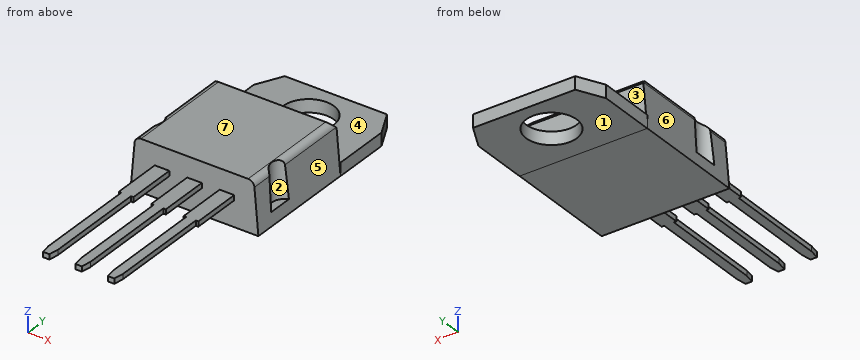
```python
from build123d import *

# Parameters (mm, degrees)
SKETCH2_W                = 10
SKETCH2_H                = 9
BOSS_EXTRUDE1_DEPTH      = 4
CHAMFER1_SIZE            = 0.5
CUT_EXTRUDE1_DEPTH       = 3
BOSS_EXTRUDE2_DEPTH      = 0.4
LPATTERN1_COUNT          = 2
LPATTERN1_PITCH          = 2.54
LPATTERN2_COUNT          = 2
LPATTERN2_PITCH          = 2.54
DRAFT2_ANGLE             = -5
BOSS_EXTRUDE3_DEPTH      = 0.01
BOSS_EXTRUDE3_DEPTH_BACK = 1
SKETCH8_R                = 1.98
FILLET1_R                = 0.5
SCALE1_SCALE             = 0.6


with BuildPart() as part:
    # Sketch2 → Boss-Extrude1 (new body)
    with BuildSketch(Plane.XY):
        Rectangle(SKETCH2_W, SKETCH2_H)
    extrude(amount=BOSS_EXTRUDE1_DEPTH)

    # Chamfer1
    chamfer1_edges = [part.edges().sort_by_distance(p)[0] for p in [
        (0, 4.5, 4),
    ]]
    chamfer(chamfer1_edges, length=CHAMFER1_SIZE)

    # Sketch6 → Cut-Extrude1 (cut)
    with BuildSketch(Plane.XY.offset(4)):
        with BuildLine():
            Line((5, -1), (5, -3))
            ThreePointArc((5, -3), (4.25, -2), (5, -1))
        make_face()
    cut_extrude1 = extrude(amount=-CUT_EXTRUDE1_DEPTH, mode=Mode.SUBTRACT)

    # Mirror1: Cut-Extrude1 across plane
    add(cut_extrude1.mirror(Plane(origin=(0, 0, 0), x_dir=(0, 0, 1), z_dir=(1, 0, 0))), mode=Mode.SUBTRACT)

    # Sketch7 → Boss-Extrude2 (add)
    with BuildSketch(Plane.XY.offset(2)):
        Polygon((-0.57, -4.5), (-0.57, -8.44), (-0.375, -8.44), (-0.375, -16.44), (-0.25, -17.2), (0.25, -17.2), (0.375, -16.44), (0.375, -8.44), (0.57, -8.44), (0.57, -4.5), align=None)
    boss_extrude2 = extrude(amount=BOSS_EXTRUDE2_DEPTH)

    # LPattern1: Boss-Extrude2 ×2
    with Locations(*[(-i * LPATTERN1_PITCH, 0, 0) for i in range(1, LPATTERN1_COUNT)]):
        add(boss_extrude2)

    # LPattern2: Boss-Extrude2 ×2
    with Locations(*[(i * LPATTERN2_PITCH, 0, 0) for i in range(1, LPATTERN2_COUNT)]):
        add(boss_extrude2)

    # Draft2
    draft2_faces = [part.faces().sort_by_distance(p)[0] for p in [
        (5, 0.383542538, 1.891910739),
        (-5, 0.383542538, 1.891910739),
    ]]
    draft(draft2_faces, Plane(origin=(0, 0, 0), x_dir=(-1, 0, 0), z_dir=(0, 0, -1)), DRAFT2_ANGLE)

    # Sketch8 → Boss-Extrude3 (add, two sides: drawn at the far end of the back side and taken through both)
    with BuildSketch(Plane(origin=(0, 0, 0), x_dir=(-1, 0, 0), z_dir=(0, 0, -1)).offset(-BOSS_EXTRUDE3_DEPTH_BACK)):
        Polygon((-5, 9), (-4, 11), (4, 11), (5, 9), (5, 4.5), (-5, 4.5), align=None)
        with Locations(Location((0, 8, 0), (0, 0, 180))):
            Circle(SKETCH8_R, mode=Mode.SUBTRACT)
    extrude(amount=BOSS_EXTRUDE3_DEPTH + BOSS_EXTRUDE3_DEPTH_BACK)

    # Fillet1
    fillet1_edges = [part.edges().sort_by_distance(p)[0] for p in [
        (-4.650045346, 1.410302183, 4),
        (4.650045346, 1.410302183, 4),
    ]]
    fillet(fillet1_edges, radius=FILLET1_R)


with BuildPart() as part_1:
    # Scale1: scaled about (0, 0, 0)
    add(part.part.scale(SCALE1_SCALE))


solid = part_1.part
```
Geometry check sheet. Reference: the model listing, model coordinates, mm. Face numbers are marked on the shaded views. A direction names the side the tool comes from. Give positions to 0.01 mm unless a question says otherwise; leave off trailing zeros. Write each loop counter-clockwise with the first axis right and the second up, starting at its lowest first coordinate (ties: lowest second). Pieces come first, ordered by that corner, then holes.
1) Access from +Z, -Z, +X, -X, +Y, -Y to the whole of each face (thin tool, end or side, straight path). Record for the marked faces 4, 5, 6 and 7.
2) Section check B-B, the plane y = -4.25. Record the boundary of the cut face in (x, z).
3) Release check for a two-part mould opening along Y. For the marked faces 1, 2 and 3 record: pulls with the +Y half, pulls with the -Y half, needs draft (parallel to the pull), parting line crosses it, or undercut.
4) Material ranges on L1, parallel to X at y = -6.25, z = 1.3 (3 decimals); L2, parallel to X at y = 4.8, z = 0.25; L3, parallel to Y at x = 0, z = 0.5, recorded low to high.
5) Gauge pin test, flat ends, axial feed: pin 1 (3 mm diameter, centred on x = 0, y = 4.8, fed in from +Z); pin 2 (0.8 mm diameter, centred on x = 0, y = -8, fed in from -Z); pin 3 (0.8 mm diameter, centred on x = -1.5, y = -5.5, fed in from +Z). Record the tip position at first contact, or that the pin passes through.
6) Section check C-C, the plane y = 4.8. Record the boundary of the cut face in (x, z), and give its area (3 significant figures).
Computed:
1. face 4: +Z, +X, -X, +Y
1. face 5: +Z, +X, -Y
1. face 6: +Z, -X, -Y
1. face 7: +Z, +X, -X, +Y, -Y
2. outline: (-1.87, 1.2) - (-1.18, 1.2) - (-1.18, 1.44) - (-1.87, 1.44) - close; (-0.34, 1.2) - (0.34, 1.2) - (0.34, 1.44) - (-0.34, 1.44) - close; (1.18, 1.2) - (1.87, 1.2) - (1.87, 1.44) - (1.18, 1.44) - close
3. face 1: needs draft
3. face 2: undercut
3. face 3: pulls with the +Y half
4. L1: x = -1.749 to -1.299, -0.225 to 0.225, 1.299 to 1.749
4. L2: x = -3 to -1.19, 1.19 to 3
4. L3: y = -2.7 to 3.61, 5.99 to 6.6
5. pin 1: stops at z = 0.6
5. pin 2: stops at z = 1.2
5. pin 3: stops at z = 1.44
6. outline: (-3, -0.01) - (-1.19, -0.01) - (-1.19, 0.6) - (-3, 0.6) - close; (1.19, -0.01) - (3, -0.01) - (3, 0.6) - (1.19, 0.6) - close
6. area: 2.20 mm2
